Autodesk Inventor part; units mm, degrees
ref_plane "YZ Plane" through (0, 0, 0) normal (1, 0, 0) x (0, 1, 0)
ref_plane "XZ Plane" through (0, 0, 0) normal (0, 1, 0) x (-1, 0, 0)
ref_plane "XY Plane" through (0, 0, 0) normal (0, 0, 1) x (1, 0, 0)
sketch "Sketch1" plane through (0, 0, 0) normal (0, 0, 1) x (1, 0, 0)
  line L0 (-190.5, 76.2) -> (-190.5, 0)
  line L1 (-190.5, 0) -> (190.5, 0)
  line L2 (190.5, 0) -> (190.5, 76.2)
  line L3 (190.5, 76.2) -> (120.6918, 76.2)
  line L4 (-190.5, 76.2) -> (-120.6918, 76.2)
  arc A0 (-120.6918, 76.2) -> (120.6918, 76.2) centre (0, 184.15) ccw
  point P0 (0, 0)
  point P1 (0, 0)
  dimension "d0" = 161.925
  dimension "d1" = 381
  dimension "d2" = 190.5
  dimension "d3" = 76.2
  dimension "d4" = 184.15
extrude "Extrusion1" add sketch "Sketch1" along normal mid plane 25.4
sketch "Sketch2" plane through (-190.5, 76.2, 12.7) normal (0, 1, 0) x (1, 0, 0)
  line L0 (0, 25.4) -> (69.8082, 0) construction
  line L1 (69.8082, 0) -> (0, 0)
  line L2 (69.8082, 25.4) -> (69.8082, 0)
  line L3 (0, 0) -> (0, 25.4)
  line L4 (0, 25.4) -> (69.8082, 25.4)
  line L5 (0, 0) -> (69.8082, 25.4) construction
  point P0 (53.9541, 12.7)
  point P1 (34.9041, 12.7)
  dimension "d14" = 19.05
hole "Hole1" at (-136.5459, 76.2, 0) direction (0, -1, 0) diameter 8.89 end through all counterbore diameter 15.24 counterbore depth 27.94
sketch "Sketch3" plane through (0, 0, 12.7) normal (0, 0, 1) x (1, 0, 0)
  line L0 (-120.6918, 76.2) -> (-190.5, 76.2)
  line L1 (-190.5, 76.2) -> (-190.5, 0)
  point P0 (0, 0)
  point P1 (-165.1, 50.8)
  dimension "d23" = 25.4
  dimension "d24" = 25.4
hole "Hole2" at (-165.1, 50.8, 12.7) direction (0, 0, -1) diameter 25.4 end through all
mirror "Mirror1" about plane through (0, 0, 0) normal (1, 0, 0) of "Hole1", "Hole2"
properties part number "Tank Holder"
Here's how the part is built. I have some questions about the finished solid (model axes, mm). A direction names the side the tool comes from. Give positions to 0.01 mm unless a question says otherwise; leave off trailing zeros. Loops run counter-clockwise (first coordinate to the right, second up) from the corner with the lowest first, then second, coordinate; pieces in that order, holes last. Notation, with made-up numbers: M -4,25 L 24,25 A10 ccw 24,44 Z; hole C 56,33 d2. An arc over 180 degrees is marked long. Use one line per item in the form item = value. Start each with the question number.
Q1. If we section it at B-B (x = -165.1): Write out the boundary of the cut face in (y, z), then the cut area to 3 significant figures.
Q2. If we section it at D-D (y = 56.5): Write out the boundary of the cut face in (x, z).
Q3. Thinking about a two-plate mould opening in Z: for faces 1 (the flat face through (-133, 48.26, 3)), 2 (the flat face through (133, 48.26, -3)), 3 (the cylindrical face through (-175.809, 43.973, -0.178)), 4 (the flat face through (-3, 22, -12.7)), which applies, +Z half, -Z half, draft (parallel to the pull), parting line (faces both ways), or undercut?
Q4. If we section it at A-A (z = 0): Write out the boundary of the cut face in (x, y).
Q5. I need wall thicknesses on line 1 along Y through (x, z) = (165.1, -5.5); line 2 along X through (y, z) = (59.5, 0); line 3 along X through (y, z) = (60.5, 0). Which ranges of each line are inside material? Lowest first, please.
Q6. Will this pin go through, and if not, where does the flat tip stop? pin 1 Ø5.5 at (x, z) = (136.55, 0) entering from -Y.
Q7. If we section it at C-C (y = 27.5): Write out the boundary of the cut face in (x, z) (3 decimals).
Q8. Which directions (+Z, -Z, +X, -X, +Y, -Y) give clear straight access to the entire face, cutting with the end or side of a thin tool? Please do faces 5 (the cylindrical face through (143.985, 62.034, -1.652)), 6 (the flat face through (-3, 22, 12.7)).
Taken from the geometry:
q1.outline = M 0,-12.7 L 38.1,-12.7 L 38.1,12.7 L 0,12.7 Z; M 63.5,-12.7 L 76.2,-12.7 L 76.2,12.7 L 63.5,12.7 Z
q1.area = 1,290 mm^2
q2.outline = M -190.5,-12.7 L -176.45,-12.7 L -176.45,12.7 L -190.5,12.7 Z; M -153.75,-12.7 L -99.63,-12.7 L -99.63,12.7 L -153.75,12.7 Z; M 99.63,-12.7 L 153.75,-12.7 L 153.75,12.7 L 99.63,12.7 Z; M 176.45,-12.7 L 190.5,-12.7 L 190.5,12.7 L 176.45,12.7 Z; hole C -136.55,0 d15.24; hole C 136.55,0 d15.24
q3.face_1 = undercut
q3.face_2 = undercut
q3.face_3 = draft
q3.face_4 = -Z half
q4.outline = M -190.5,0 L -140.99,0 L -140.99,48.26 L -144.17,48.26 L -144.17,76.2 L -190.5,76.2 Z; M -132.1,0 L 132.1,0 L 132.1,48.26 L 128.93,48.26 L 128.93,76.2 L 120.69,76.2 A161.93 cw -120.69,76.2 L -128.93,76.2 L -128.93,48.26 L -132.1,48.26 Z; M 140.99,0 L 190.5,0 L 190.5,76.2 L 144.17,76.2 L 144.17,48.26 L 140.99,48.26 Z; hole C -165.1,50.8 d25.4; hole C 165.1,50.8 d25.4
q5.line_1 = 0 to 38.1, 63.5 to 76.2
q5.line_2 = -190.5 to -174.35, -155.85 to -144.17, -128.93 to -103.35, 103.35 to 128.93, 144.17 to 155.85, 174.35 to 190.5
q5.line_3 = -190.5 to -173.3, -156.9 to -144.17, -128.93 to -104.55, 104.55 to 128.93, 144.17 to 156.9, 173.3 to 190.5
q6.pin_1 = through
q7.outline = M -190.5,-12.7 L -40.994,-12.7 L -40.994,12.7 L -190.5,12.7 Z; M 40.994,-12.7 L 190.5,-12.7 L 190.5,12.7 L 40.994,12.7 Z; hole C -136.546,0 d8.89; hole C 136.546,0 d8.89
q8.face_5 = +Y
q8.face_6 = +Z, +X, -X, +Y, -Y
